Autodesk Inventor part; units mm, degrees
ref_plane "YZ Plane" through (0, 0, 0) normal (1, 0, 0) x (0, 1, 0)
ref_plane "XZ Plane" through (0, 0, 0) normal (0, 1, 0) x (-1, 0, 0)
ref_plane "XY Plane" through (0, 0, 0) normal (0, 0, 1) x (1, 0, 0)
sketch "Sketch1" plane through (0, 0, 0) normal (0, 0, 1) x (1, 0, 0)
  line L0 (-14.1, -15.1) -> (14.1, -15.1)
  line L1 (14.1, -15.1) -> (14.1, 15.1)
  line L2 (14.1, 15.1) -> (-14.1, 15.1)
  line L3 (-14.1, 15.1) -> (-14.1, -15.1)
  line L4 (-14.1, -15.1) -> (14.1, 15.1) construction
  line L5 (14.1, -15.1) -> (-14.1, 15.1) construction
  line L6 (-114.9, -114.9) -> (114.9, -114.9)
  line L7 (114.9, -114.9) -> (114.9, 114.9)
  line L8 (114.9, 114.9) -> (-114.9, 114.9)
  line L9 (-114.9, 114.9) -> (-114.9, -114.9)
  line L10 (-114.9, -114.9) -> (114.9, 114.9) construction
  line L11 (114.9, -114.9) -> (-114.9, 114.9) construction
  line L12 (-114.9, -114.9) -> (114.9, -114.9)
  line L13 (114.9, -114.9) -> (114.9, -64.9)
  line L14 (114.9, -64.9) -> (-114.9, -64.9)
  line L15 (-114.9, -64.9) -> (-114.9, -114.9)
  point P0 (0, 0)
  point P1 (-114.9, -64.9)
  dimension "d0" = 28.2
  dimension "d1" = 30.2
  dimension "d2" = 229.8
  dimension "d3" = 229.8
  dimension "d4" = 179.8
  dimension "d9" = 64.9
  dimension "d10" = 114.9
extrude "Extrusion1" add sketch "Sketch1" along normal blind 3 contours L9 L8 L7 L14
fillet "Fillet1" radius 3 4 edges at (-14.1, -15.1, 1.5) (-14.1, 15.1, 1.5) (14.1, 15.1, 1.5) (14.1, -15.1, 1.5)
fillet "Fillet2" radius 3 4 edges at (114.9, 114.9, 1.5) (114.9, -64.9, 1.5) (-114.9, -64.9, 1.5) (-114.9, 114.9, 1.5)
properties part number "ChamberCamSide"
Here's how the part is built. I have some questions about the finished solid (model axes, mm). Coordinates: 2 decimals unless noted, no trailing zeros. Write each loop counter-clockwise with the first axis right and the second up, starting at its lowest first coordinate (ties: lowest second). Pieces come first, ordered by that corner, then holes. Notation, with made-up numbers: (-1, 88) - (56, 88) arc R14 ccw to (56, 115) - close; hole circle Ø2 at (45, 86). An arc over 180 degrees is marked (long way). One line per item, written item: value.
1) Suppose I cut it at A-A on y = 2.5. Write out the boundary of the cut face in (x, z).
Model answer:
outline: (-114.9, 0) - (-14.1, 0) - (-14.1, 3) - (-114.9, 3) - close; (14.1, 0) - (114.9, 0) - (114.9, 3) - (14.1, 3) - close
2) I need wall thicknesses on line 1 along Y through (x, z) = (-8, 1.05); line 2 along X through (y, z) = (-5, 2.45); line 3 along X through (y, z) = (-14.5, 1.25). Which ranges of each line are inside material? Lowest first, please.
Model answer:
line 1: y = -64.9 to -15.1, 15.1 to 114.9
line 2: x = -114.9 to -14.1, 14.1 to 114.9
line 3: x = -114.9 to -12.9, 12.9 to 114.9
3) Suppose I cut it at B-B on z = 1.65. Write out the boundary of the cut face in (x, y), and give its area (3 significant figures).
Model answer:
outline: (-114.9, -61.9) arc R3 ccw to (-111.9, -64.9) - (111.9, -64.9) arc R3 ccw to (114.9, -61.9) - (114.9, 111.9) arc R3 ccw to (111.9, 114.9) - (-111.9, 114.9) arc R3 ccw to (-114.9, 111.9) - close; hole (-14.1, -12.1) arc R3 ccw to (-11.1, -15.1) - (11.1, -15.1) arc R3 ccw to (14.1, -12.1) - (14.1, 12.1) arc R3 ccw to (11.1, 15.1) - (-11.1, 15.1) arc R3 ccw to (-14.1, 12.1) - close
area: 40,500 mm²
